Input: part model. Units: mm. Frame: model coordinates. Give positions to 0.01 mm unless a question says otherwise; leave off trailing zeros. Loops run counter-clockwise (first coordinate to the right, second up) from the corner with the lowest first, then second, coordinate; pieces in that order, holes last. Notation, with made-up numbers: (14.5, -39) -> (53.5, -39) arc R26 ccw to (53.5, -4) -> close; hole circle Ø4 at (32.5, -40). An arc over 180 degrees is marked (long way). Answer in a Markdown table with one row per item. Add a question column.
```python
from build123d import *

# Parameters (mm, degrees)
SKIZZE1_W                                            = 50
SKIZZE1_H                                            = 30
BASIS_BLECH1_DEPTH                                   = 1.5
VERRUNDUNG1_R                                        = 5
FORMSENKUNG_F_R_M3_SENKSCHRAUBE_MIT_INNE_D           = 1.6
FORMSENKUNG_F_R_M3_SENKSCHRAUBE_MIT_INNE_DEPTH       = 8
FORMSENKUNG_F_R_M3_SENKSCHRAUBE_MIT_INNE_CSINK_D     = 3.5
FORMSENKUNG_F_R_M3_SENKSCHRAUBE_MIT_INNE_CSINK_ANGLE = 90
FORMSENKUNG_F_R_M3_SENKSCHRAUBE_MIT_INNE_TIP         = 0.480688495
SKIZZE8_R                                            = 1
SCHNITT_LINEAR_AUSTRAGEN1_DEPTH                      = 30.193321154


# Sheet-metal steps are written as plain solids
with BuildPart() as part:
    # Skizze1 → Basis-Blech1 (new body)
    with BuildSketch(Plane.XY):
        Rectangle(SKIZZE1_W, SKIZZE1_H)
    extrude(amount=-BASIS_BLECH1_DEPTH)

    # Verrundung1
    verrundung1_edges = [part.edges().sort_by_distance(p)[0] for p in [
        (-25, 15, -0.75),
        (25, 15, -0.75),
        (25, -15, -0.75),
        (-25, -15, -0.75),
    ]]
    fillet(verrundung1_edges, radius=VERRUNDUNG1_R)

    # Formsenkung für M3 Senkschraube mit Innensechskant2
    with Locations(Plane(origin=(-12.308549643, 4.902846213, 0), x_dir=(-1, 0, 0), z_dir=(0, 0, 1))):
        with Locations((-32.308549643, -1.097153787), (-12.308549643, -7.097153787), (7.691450357, -1.097153787), (7.691450357, 10.902846213), (-12.308549643, 16.902846213), (-32.308549643, 10.902846213)):
            CounterSinkHole(FORMSENKUNG_F_R_M3_SENKSCHRAUBE_MIT_INNE_D / 2, FORMSENKUNG_F_R_M3_SENKSCHRAUBE_MIT_INNE_CSINK_D / 2, depth=FORMSENKUNG_F_R_M3_SENKSCHRAUBE_MIT_INNE_DEPTH, counter_sink_angle=FORMSENKUNG_F_R_M3_SENKSCHRAUBE_MIT_INNE_CSINK_ANGLE)
            with Locations((0, 0, -(FORMSENKUNG_F_R_M3_SENKSCHRAUBE_MIT_INNE_DEPTH + FORMSENKUNG_F_R_M3_SENKSCHRAUBE_MIT_INNE_TIP / 2))):  # 118° drill point
                Cone(0, FORMSENKUNG_F_R_M3_SENKSCHRAUBE_MIT_INNE_D / 2, FORMSENKUNG_F_R_M3_SENKSCHRAUBE_MIT_INNE_TIP, mode=Mode.SUBTRACT)

    # Skizze8 → Schnitt-Linear austragen1 (cut, through all)
    with BuildSketch(Plane(origin=(0, 0, -1.5), x_dir=(-1, 0, 0), z_dir=(0, 0, -1))):
        with Locations((-20, 6)):
            Circle(SKIZZE8_R)
        with Locations((0, 12)):
            Circle(SKIZZE8_R)
        with Locations((20, 6)):
            Circle(SKIZZE8_R)
        with Locations((20, -6)):
            Circle(SKIZZE8_R)
        with Locations((0, -12)):
            Circle(SKIZZE8_R)
        with Locations((-20, -6)):
            Circle(SKIZZE8_R)
    extrude(amount=-SCHNITT_LINEAR_AUSTRAGEN1_DEPTH, mode=Mode.SUBTRACT)


solid = part.part
```
1) Pin query (flat end, axial travel): pin 1 (2.5 mm diameter, centred on x = -20, y = 6, fed in from +Z). Return the tip coordinate at first contact, or that it passes through.
2) Material intervals for line 1 along Y through (x, z) = (0, -1); line 2 along Y through (x, z) = (-20, -0.85); line 3 along X through (y, z) = (-6, -1.15), sorted ascending.
3) Section A-A on y = -6. Output: boundary loops of the cut face in (x, z).
4) Pull-direction query (X, two-part tool) for faces 1 (the face through (-24, -13, -1)), 2 (the face through (0, -15, -1)), 3 (the face through (0, -11, -1)); classes: +X half, -X half, draft (parallel to the pull), parting line (faces both ways), or undercut.
5) Section B-B on x = 0. Output: boundary loops of the cut face in (y, z).
6) Section C-C on z = -0.5. Output: boundary loops of the cut face in (x, y), and give its area (3 significant figures).
7) Section D-D on y = -12. Output: boundary loops of the cut face in (x, z), and give its area (3 significant figures).
Working result:
| question | item | result |
|---|---|---|
| 1 | pin 1 | stops at z = -0.5 |
| 2 | line 1 | y = -15 to -13, -11 to 11, 13 to 15 |
| 2 | line 2 | y = -15 to -7, -5 to 5, 7 to 15 |
| 2 | line 3 | x = -25 to -21, -19 to 19, 21 to 25 |
| 3 | outline | (-25, -1.5) -> (-21, -1.5) -> (-21, -0.75) -> (-21.75, 0) -> (-25, 0) -> close; (-19, -1.5) -> (19, -1.5) -> (19, -0.75) -> (18.25, 0) -> (-18.25, 0) -> (-19, -0.75) -> close; (21, -1.5) -> (25, -1.5) -> (25, 0) -> (21.75, 0) -> (21, -0.75) -> close |
| 4 | face 1 | -X half |
| 4 | face 2 | draft |
| 4 | face 3 | undercut |
| 5 | outline | (-15, -1.5) -> (-13, -1.5) -> (-13, -0.75) -> (-13.75, 0) -> (-15, 0) -> close; (-11, -1.5) -> (11, -1.5) -> (11, -0.75) -> (10.25, 0) -> (-10.25, 0) -> (-11, -0.75) -> close; (13, -1.5) -> (15, -1.5) -> (15, 0) -> (13.75, 0) -> (13, -0.75) -> close |
| 6 | outline | (-25, -10) arc R5 ccw to (-20, -15) -> (20, -15) arc R5 ccw to (25, -10) -> (25, 10) arc R5 ccw to (20, 15) -> (-20, 15) arc R5 ccw to (-25, 10) -> close; hole circle Ø2.5 at (-20, -6); hole circle Ø2.5 at (-20, 6); hole circle Ø2.5 at (0, -12); hole circle Ø2.5 at (0, 12); hole circle Ø2.5 at (20, -6); hole circle Ø2.5 at (20, 6) |
| 6 | area | 1,450 mm2 |
| 7 | outline | (-24.58, -1.5) -> (-1, -1.5) -> (-1, -0.75) -> (-1.75, 0) -> (-24.58, 0) -> close; (1, -1.5) -> (24.58, -1.5) -> (24.58, 0) -> (1.75, 0) -> (1, -0.75) -> close |
| 7 | area | 70.2 mm2 |
